from build123d import *

# Parameters (mm, degrees)
F0_R     = 6
F1_DEPTH = 24
F3_D     = 4.2
F3_DEPTH = 14.4
F3_TIP   = 1.2618073
F5_D     = 2.5
F5_DEPTH = 5
F5_START = 0.1316528
F5_TIP   = 0.7510757738


with BuildPart() as f1:
    # F0 (on Front) → F1 (new body)
    with BuildSketch(Plane.XZ):
        with BuildLine():
            Line((8, 12.7148411355), (-8, 12.7148411355))
            Line((-8, 12.7148411355), (-8, -9))
            ThreePointArc((-8, -9), (-6.2426406871, -13.2426406871), (-2, -15))
            Line((-2, -15), (2, -15))
            ThreePointArc((2, -15), (6.2426406871, -13.2426406871), (8, -9))
            Line((8, -9), (8, 12.7148411355))
        make_face()
        with Locations((0, -6)):
            Circle(F0_R, mode=Mode.SUBTRACT)
    extrude(amount=-F1_DEPTH)

    # F3
    with Locations(Plane.XY.offset(12.7148411355)):
        with Locations((0, 18), (0, 6)):
            Hole(F3_D / 2, depth=F3_DEPTH)
            with Locations((0, 0, -(F3_DEPTH + F3_TIP / 2))):  # 118° drill point
                Cone(0, F3_D / 2, F3_TIP, mode=Mode.SUBTRACT)

    # F5
    # its depths count from where the whole tool has entered the part; down to there all is cleared
    with Locations(Plane(origin=(-8, 0, 0), x_dir=(0, -1, 0), z_dir=(-1, 0, 0)).offset(-F5_START)):
        with Locations((-12, -9)):
            Hole(F5_D / 2, depth=F5_DEPTH)
            with Locations((0, 0, -(F5_DEPTH + F5_TIP / 2))):  # 118° drill point
                Cone(0, F5_D / 2, F5_TIP, mode=Mode.SUBTRACT)


solid = f1.part
Check sheet for the modelled part. Datum: model origin and axes. Units: mm. A direction names the side the tool comes from. Give positions to 0.01 mm unless a question says otherwise; leave off trailing zeros. Loops run counter-clockwise (first coordinate to the right, second up) from the corner with the lowest first, then second, coordinate; pieces in that order, holes last. Notation, with made-up numbers: M 36.25,87 L 82.25,87 A19 cw 82.25,94 Z; hole C 63.25,-11 d6. An arc over 180 degrees is marked long. Use a Markdown table: item, result. Add a question column.
Q1. Sectioned sample at A-A, the plane z = -6. Record the cut outline in (x, y), then the cut area to 3 significant figures.
Q2. Sectioned sample at D-D, the plane z = 3.5. Record the cut outline in (x, y).
Q3. Scan lines: line 1 along Y through (x, z) = (0, 6); line 2 along Y through (x, z) = (-6.3, -9); line 3 along X through (y, z) = (18, 9.25). Record each from-to range of solid material in increasing order. Write a range as [from, to].
Q4. Sectioned sample at B-B, the plane y = 21. Record the cut outline in (x, z), then the cut area to 3 significant figures.
Q5. Mould release check, pull along Z, two halves, no side actions. Record for faces 3 (the cylindrical face through (2.769, 11.832, -11.323)), 4 (the flat face through (0, 12, 12.715)), 5 (the cylindrical face through (-6.51, 11.73, -10.22)), 6 (the flat face through (0, 12, -15)): pulls with the +Z half, pulls with the -Z half, needs draft (parallel to the pull), parting line crosses it, or undercut.
Q6. Tool access check on faces 1 (the cylindrical face through (-1.13, 19.77, 6.08)), 2 (the flat face through (0, 0, 2)). Record the directions out of +Z, -Z, +X, -X, +Y, -Y that give a thin tool (end or side, any length) a straight path to the whole face; none if there is none.
Q7. Go/stop test with a flat-tipped pin: pin 1 (4 mm diameter, centred on x = 5, y = 4, fed in from -Z). Record where the tip stops, or that it passes through.
Q8. Sectioned sample at C-C, the plane x = 0. Record the cut outline in (y, z).
Verdict:
| question | item | result |
|---|---|---|
| 1 | outline | M -8,0 L -6,0 L -6,24 L -8,24 Z; M 6,0 L 8,0 L 8,24 L 6,24 Z |
| 1 | area | 96.0 mm^2 |
| 2 | outline | M -8,0 L 8,0 L 8,24 L -8,24 Z; hole C 0,6 d4.2; hole C 0,18 d4.2 |
| 3 | line 1 | [0, 3.9], [8.1, 15.9], [20.1, 24] |
| 3 | line 2 | [0, 10.75], [13.25, 24] |
| 3 | line 3 | [-8, -2.1], [2.1, 8] |
| 4 | outline | M -8,-9 A6 ccw -2,-15 L 2,-15 A6 ccw 8,-9 L 8,12.71 L -8,12.71 Z; hole C 0,-6 d12 |
| 4 | area | 315 mm^2 |
| 5 | face 3 | undercut |
| 5 | face 4 | pulls with the +Z half |
| 5 | face 5 | undercut |
| 5 | face 6 | pulls with the -Z half |
| 6 | face 1 | +Z |
| 6 | face 2 | +Z, -Z, +X, -X, -Y |
| 7 | pin 1 | z = -14.92 |
| 8 | outline | M 0,-15 L 24,-15 L 24,-12 L 0,-12 Z; M 0,0 L 3.9,0 L 3.9,12.71 L 0,12.71 Z; M 8.1,0 L 15.9,0 L 15.9,12.71 L 8.1,12.71 Z; M 20.1,0 L 24,0 L 24,12.71 L 20.1,12.71 Z |
